from build123d import *

# Parameters (mm, degrees)
F0_W     = 83.4
F0_H     = 44.6
F1_DEPTH = 9
F2_DEPTH = 10
F0_W_2   = 4
F0_H_2   = 40.6
F3_DEPTH = 4
F4_D     = 4
F4_DEPTH = 15
F4_TIP   = 1.2017212381
F5_R     = 5
F6_R     = 1


with BuildPart() as f1:
    # F0 (on Top) → F1 (new body)
    with BuildSketch(Plane.XY):
        Rectangle(F0_W, F0_H)
        Polygon((-39.7, -20.3), (-39.7, 20.3), (-2, 20.3), (2, 20.3), (39.7, 20.3), (39.7, -20.3), (2, -20.3), (-2, -20.3), align=None, mode=Mode.SUBTRACT)
    extrude(amount=F1_DEPTH)

    # F0 (on Top) → F2 (join)
    with BuildSketch(Plane.XY):
        Polygon((-5, 25.3), (-44.7, 25.3), (-44.7, -25.3), (-5, -25.3), (5, -25.3), (44.7, -25.3), (44.7, 25.3), (5, 25.3), align=None)
        Rectangle(F0_W, F0_H, mode=Mode.SUBTRACT)
        with BuildLine():
            Line((5, -25.3), (-5, -25.3))
            ThreePointArc((-5, -25.3), (0, -30.3), (5, -25.3))
        make_face()
        with BuildLine():
            ThreePointArc((5, 25.3), (0, 30.3), (-5, 25.3))
            Line((-5, 25.3), (5, 25.3))
        make_face()
    extrude(amount=F2_DEPTH)

    # F0 (on Top) → F3 (join)
    with BuildSketch(Plane.XY):
        Rectangle(F0_W_2, F0_H_2)
    extrude(amount=F3_DEPTH)

    # F4
    with Locations(Plane(origin=(0, 0, 0), x_dir=(1, 0, 0), z_dir=(0, 0, -1))):
        with Locations((0, -25.3), (0, 25.3)):
            Hole(F4_D / 2, depth=F4_DEPTH)
            with Locations((0, 0, -(F4_DEPTH + F4_TIP / 2))):  # 118° drill point
                Cone(0, F4_D / 2, F4_TIP, mode=Mode.SUBTRACT)

    # F5
    f5_edges = [f1.edges().sort_by_distance(p)[0] for p in [
        (-44.7, 25.3, 5),
        (-5, 25.3, 5),
        (5, 25.3, 5),
        (44.7, 25.3, 5),
        (44.7, -25.3, 5),
        (-5, -25.3, 5),
        (5, -25.3, 5),
        (-44.7, -25.3, 5),
        (2, 20.3, 2),
        (-2, 20.3, 2),
        (2, -20.3, 2),
        (-2, -20.3, 2),
        (39.7, 20.3, 4.5),
        (-39.7, 20.3, 4.5),
        (-39.7, -20.3, 4.5),
        (39.7, -20.3, 4.5),
    ]]
    fillet(f5_edges, radius=F5_R)

    # F6
    f6_edges = [f1.edges().sort_by_distance(p)[0] for p in [
        (-43.235534, 23.835534, 10),
    ]]
    fillet(f6_edges, radius=F6_R)


solid = f1.part
The model under review builds one solid part; all positions refer to its coordinate system, in mm. A direction names the side the tool comes from. Round coordinates to 2 decimals unless told otherwise and drop trailing zeros. Loops run counter-clockwise (first coordinate to the right, second up) from the corner with the lowest first, then second, coordinate; pieces in that order, holes last. Notation, with made-up numbers: (48.5, 51.25) -> (52.5, 51.25) arc R21 ccw to (52.5, 74.25) -> close; hole circle Ø3 at (-16, 31). An arc over 180 degrees is marked (long way). Write item = value, one per line. Start each with the question number.
Item 1: For faces 1 (the flat face through (-24, -25.3, 4)), 2 (the flat face through (24, -25.3, 4)), 3 (the flat face through (-1, 0, 4)), 4 (the cylindrical face through (38.2, 18.87, 4.56)), list the 3-axis set-ups (+Z, -Z, +X, -X, +Y, -Y) from which the entire face can be reached by the end or side of a thin tool; tool diameter is ignored.
Item 2: To check wall thickness, follow L1, parallel to X at y = 4, z = 3.75; L2, parallel to X at y = 18.5, z = 2.75; L3, parallel to Y at x = -18, z = 7.5. State the ranges of each line that lie inside material, in increasing order.
Item 3: Mouldability with a two-part tool opening along X and no side actions: class faces 5 (the cylindrical face through (-43.27, 23.8, 4.56)), 6 (the cylindrical face through (3.5, 18.87, 2.03)), 7 (the flat face through (24, 25.3, 4)) as released by +X, released by -X, zero draft, split by the parting line, or undercut.
Item 4: Take a section at B-B on y = 12.5. Give the boundary of the cut face in (x, z), plus the area to 3 significant figures.
Item 5: Take a section at C-C on x = -32. Give the boundary of the cut face in (y, z).
Item 6: Insertion check: pin 1 (0.8 mm diameter, centred on y = -4.5, z = 9.5, fed in from -X) (3 decimals); pin 2 (1.1 mm diameter, centred on x = 10, z = 9.5, fed in from -Y); pin 3 (4 mm diameter, centred on x = -3, z = 8.5, fed in from +Y). Each pin has a flat end and moves straight along its axis. Give the tip position at first contact, or say it passes through.
Item 7: Take a section at D-D on z = 6.5. Give the boundary of the cut face in (x, y).
Item 8: Take a section at A-A on x = 0. Give the boundary of the cut face in (y, z), plus the area to 3 significant figures.
Result:
q1.face_1 = +Z, -Z, -X, -Y
q1.face_2 = +Z, -Z, +X, -Y
q1.face_3 = +Z
q1.face_4 = +Z, -Z
q2.L1 = -44.7 to -39.7, -2 to 2, 39.7 to 44.7
q2.L2 = -44.7 to -38.54, -3.16 to 3.16, 38.54 to 44.7
q2.L3 = -25.3 to -20.3, 20.3 to 25.3
q3.face_5 = released by -X
q3.face_6 = undercut
q3.face_7 = zero draft
q4.outline = (-44.7, 0) -> (-39.7, 0) -> (-39.7, 9) -> (-41.7, 9) -> (-41.7, 10) -> (-43.7, 10) arc R1 ccw to (-44.7, 9) -> close; (-2, 0) -> (2, 0) -> (2, 4) -> (-2, 4) -> close; (39.7, 0) -> (44.7, 0) -> (44.7, 9) arc R1 ccw to (43.7, 10) -> (41.7, 10) -> (41.7, 9) -> (39.7, 9) -> close
q4.area = 112 mm²
q5.outline = (-25.3, 0) -> (-20.3, 0) -> (-20.3, 9) -> (-22.3, 9) -> (-22.3, 10) -> (-24.3, 10) arc R1 ccw to (-25.3, 9) -> close; (20.3, 0) -> (25.3, 0) -> (25.3, 9) arc R1 ccw to (24.3, 10) -> (22.3, 10) -> (22.3, 9) -> (20.3, 9) -> close
q6.pin_1 = -44.695
q6.pin_2 = -25.3
q6.pin_3 = 30.2
q7.outline = (-44.7, -20.3) arc R5 ccw to (-39.7, -25.3) -> (-8.66, -25.3) arc R5 cw to (-4.33, -27.8) arc R5 ccw to (4.33, -27.8) arc R5 cw to (8.66, -25.3) -> (39.7, -25.3) arc R5 ccw to (44.7, -20.3) -> (44.7, 20.3) arc R5 ccw to (39.7, 25.3) -> (8.66, 25.3) arc R5 cw to (4.33, 27.8) arc R5 ccw to (-4.33, 27.8) arc R5 cw to (-8.66, 25.3) -> (-39.7, 25.3) arc R5 ccw to (-44.7, 20.3) -> close; hole (-39.7, -15.3) arc R5 ccw to (-34.7, -20.3) -> (34.7, -20.3) arc R5 ccw to (39.7, -15.3) -> (39.7, 15.3) arc R5 ccw to (34.7, 20.3) -> (-34.7, 20.3) arc R5 ccw to (-39.7, 15.3) -> close; hole circle Ø4 at (0, -25.3); hole circle Ø4 at (0, 25.3)
q8.outline = (-30.3, 0) -> (-27.3, 0) -> (-27.3, 10) -> (-29.3, 10) arc R1 ccw to (-30.3, 9) -> close; (-23.3, 0) -> (23.3, 0) -> (23.3, 10) -> (22.3, 10) -> (22.3, 9) -> (20.3, 9) -> (20.3, 4) -> (-20.3, 4) -> (-20.3, 9) -> (-22.3, 9) -> (-22.3, 10) -> (-23.3, 10) -> close; (27.3, 0) -> (30.3, 0) -> (30.3, 9) arc R1 ccw to (29.3, 10) -> (27.3, 10) -> close
q8.area = 278 mm²
